Geometry check sheet. Reference: the model listing, model coordinates, mm. A direction names the side the tool comes from. Give positions to 0.01 mm unless a question says otherwise; leave off trailing zeros. Order: outer loops, then holes, each group sorted by start corner. A loop starts at its lowest first (then second) coordinate and runs counter-clockwise, first axis right, second up.
```python
from build123d import *

# Parameters (mm, degrees)
SKETCH1_R                       = 85
SKETCH1_R_2                     = 80
SKETCH1_R_3                     = 75
BOSS_EXTRUDE1_DEPTH             = 150
SKETCH1_4_R                     = 80
SKETCH1_4_R_2                   = 75
CUT_EXTRUDE1_DEPTH              = 155
SKETCH2_R                       = 85
BOSS_EXTRUDE3_DEPTH             = 5
SKETCH2_3_W                     = 20
SKETCH2_3_H                     = 96
BOSS_EXTRUDE4_DEPTH             = 176
SKETCH2_4_W                     = 20
SKETCH2_4_H                     = 96
BOSS_EXTRUDE5_DEPTH             = 176
SKETCH3_R                       = 23.5
CUT_EXTRUDE3_DEPTH              = 90
CUT_EXTRUDE4_DEPTH              = 120
CUT_EXTRUDE5_DEPTH              = 20
CUT_EXTRUDE6_START              = -20
CUT_EXTRUDE6_DEPTH              = 20
SKETCH6_R                       = 2
CUT_EXTRUDE7_DEPTH              = 20
SKETCH11_R                      = 2.5
CUT_EXTRUDE10_DEPTH             = 131
SKETCH1_7_R                     = 80
SKETCH1_7_R_2                   = 75
BOSS_EXTRUDE6_DEPTH             = 155
CUT_EXTRUDE12_DEPTH             = 20
CUT_EXTRUDE12_DEPTH_BACK        = 10
SKETCH1_10_R                    = 85
SKETCH1_10_R_2                  = 80
CUT_EXTRUDE13_START             = -25
SKETCH12_R                      = 85
SKETCH12_R_2                    = 80
CUT_EXTRUDE13_DEPTH             = 25
SKETCH1_11_R                    = 75
BOSS_EXTRUDE7_DEPTH             = 5
F_5_0MM_DOWEL_HOLE1_D           = 5
F_5_0MM_DOWEL_HOLE1_DEPTH       = 5
F_5_0MM_DOWEL_HOLE1_CSINK_D     = 5.05
F_5_0MM_DOWEL_HOLE1_CSINK_ANGLE = 90
F_5_0MM_DOWEL_HOLE1_TIP         = 1.502151548
BOSS_EXTRUDE8_DEPTH             = 3
SKETCH16_R                      = 25
CUT_EXTRUDE14_DEPTH             = 1


with BuildPart() as part:
    # Sketch1 → Boss-Extrude1 (new body)
    # profile 1 of 2: a face of its own
    with BuildSketch(Plane(origin=(0, 0, 0), x_dir=(1, 0, 0), z_dir=(0, 1, 0))):
        with Locations(Location((0, 0, 0), (0, 0, 270))):
            Circle(SKETCH1_R)
        Circle(SKETCH1_R_2, mode=Mode.SUBTRACT)
    # profile 2 of 2: a face of its own
    with BuildSketch(Plane(origin=(0, 0, 0), x_dir=(1, 0, 0), z_dir=(0, 1, 0))):
        Circle(SKETCH1_R_2)
        with Locations(Location((0, 0, 0), (0, 0, 270))):
            Circle(SKETCH1_R_3, mode=Mode.SUBTRACT)
    extrude(amount=BOSS_EXTRUDE1_DEPTH)

    # Sketch1_4 → Cut-Extrude1 (cut)
    with BuildSketch(Plane(origin=(0, 0, 0), x_dir=(1, 0, 0), z_dir=(0, 1, 0))):
        with Locations(Location((0, 0, 0), (0, 0, 270))):
            Circle(SKETCH1_4_R)
        Circle(SKETCH1_4_R_2, mode=Mode.SUBTRACT)
    extrude(amount=CUT_EXTRUDE1_DEPTH, mode=Mode.SUBTRACT)

    # Sketch2 → Boss-Extrude3 (add)
    with BuildSketch(Plane(origin=(0, 150, 0), x_dir=(1, 0, 0), z_dir=(0, 1, 0))):
        with Locations(Location((0, 0, 0), (0, 0, 270))):
            Circle(SKETCH2_R)
    extrude(amount=BOSS_EXTRUDE3_DEPTH)

    # Sketch2_3 → Boss-Extrude4 (add)
    with BuildSketch(Plane(origin=(0, 150, 0), x_dir=(1, 0, 0), z_dir=(0, 1, 0))):
        with Locations((50, 0)):
            Rectangle(SKETCH2_3_W, SKETCH2_3_H)
    extrude(amount=BOSS_EXTRUDE4_DEPTH)

    # Sketch2_4 → Boss-Extrude5 (add)
    with BuildSketch(Plane(origin=(0, 150, 0), x_dir=(1, 0, 0), z_dir=(0, 1, 0))):
        with Locations((-50, 0)):
            Rectangle(SKETCH2_4_W, SKETCH2_4_H)
    extrude(amount=BOSS_EXTRUDE5_DEPTH)

    # Sketch3 → Cut-Extrude3 (cut)
    with BuildSketch(Plane(origin=(60, 0, 0), x_dir=(0, 0, -1), z_dir=(1, 0, 0))):
        with Locations((0, 278)):
            Circle(SKETCH3_R)
    extrude(amount=-CUT_EXTRUDE3_DEPTH, mode=Mode.SUBTRACT)

    # Sketch3_3 → Cut-Extrude4 (cut)
    with BuildSketch(Plane(origin=(60, 0, 0), x_dir=(0, 0, -1), z_dir=(1, 0, 0))):
        with BuildLine():
            ThreePointArc((0, 300.5), (-22.5, 278), (0, 255.5))
            Line((0, 255.5), (0, 300.5))
        make_face()
        with BuildLine():
            Line((0, 300.5), (0, 255.5))
            ThreePointArc((0, 255.5), (15.909902577, 262.090097423), (22.5, 278))
            ThreePointArc((22.5, 278), (15.909902577, 293.909902577), (0, 300.5))
        make_face()
        with BuildLine():
            ThreePointArc((0, 301.5), (-23.5, 278), (0, 254.5))
            Line((0, 254.5), (0, 255.5))
            ThreePointArc((0, 255.5), (-22.5, 278), (0, 300.5))
            Line((0, 300.5), (0, 301.5))
        make_face()
        with BuildLine():
            Line((0, 255.5), (0, 254.5))
            ThreePointArc((0, 254.5), (16.617009358, 261.382990642), (23.5, 278))
            ThreePointArc((23.5, 278), (16.617009358, 294.617009358), (0, 301.5))
            Line((0, 301.5), (0, 300.5))
            ThreePointArc((0, 300.5), (15.909902577, 293.909902577), (22.5, 278))
            ThreePointArc((22.5, 278), (15.909902577, 262.090097423), (0, 255.5))
        make_face()
    extrude(amount=-CUT_EXTRUDE4_DEPTH, mode=Mode.SUBTRACT)

    # Sketch4 → Cut-Extrude5 (cut)
    with BuildSketch(Plane(origin=(60, 0, 0), x_dir=(0, 0, -1), z_dir=(1, 0, 0))):
        with BuildLine():
            Line((-48, 326), (-48, 278))
            ThreePointArc((-48, 278), (-33.941125268, 311.941125726), (6.48e-07, 326))
            Line((6.48e-07, 326), (-48, 326))
        make_face()
        with BuildLine():
            ThreePointArc((6.48e-07, 326), (33.941125726, 311.941125268), (48, 278))
            Line((48, 278), (48, 326))
            Line((48, 326), (6.48e-07, 326))
        make_face()
    extrude(amount=-CUT_EXTRUDE5_DEPTH, mode=Mode.SUBTRACT)

    # Sketch5 → Cut-Extrude6 (cut)
    with BuildSketch(Plane.ZY.offset(60).offset(CUT_EXTRUDE6_START)):
        with BuildLine():
            Line((-48, 326), (-48, 278))
            ThreePointArc((-48, 278), (-33.941125497, 311.941125497), (0, 326))
            Line((0, 326), (-48, 326))
        make_face()
        with BuildLine():
            ThreePointArc((0, 326), (33.941125497, 311.941125497), (48, 278))
            Line((48, 278), (48, 326))
            Line((48, 326), (0, 326))
        make_face()
    extrude(amount=CUT_EXTRUDE6_DEPTH, mode=Mode.SUBTRACT)

    # Sketch6 → Cut-Extrude7 (cut)
    with BuildSketch(Plane(origin=(60, 0, 0), x_dir=(0, 0, -1), z_dir=(1, 0, 0))):
        with Locations((0, 320)):
            Circle(SKETCH6_R)
        with Locations((29.69848481, 307.69848481)):
            Circle(SKETCH6_R)
        with Locations((42, 278)):
            Circle(SKETCH6_R)
        with Locations((29.69848481, 248.30151519)):
            Circle(SKETCH6_R)
        with Locations((0, 236)):
            Circle(SKETCH6_R)
        with Locations((-29.69848481, 248.30151519)):
            Circle(SKETCH6_R)
        with Locations((-42, 278)):
            Circle(SKETCH6_R)
        with Locations((-29.69848481, 307.69848481)):
            Circle(SKETCH6_R)
    extrude(amount=-CUT_EXTRUDE7_DEPTH, mode=Mode.SUBTRACT)

    # Sketch11 → Cut-Extrude10 (cut)
    with BuildSketch(Plane(origin=(60, 0, 0), x_dir=(0, 0, -1), z_dir=(1, 0, 0))):
        with Locations((-40, 195.5)):
            Circle(SKETCH11_R)
        with Locations((40, 195.5)):
            Circle(SKETCH11_R)
    extrude(amount=-CUT_EXTRUDE10_DEPTH, mode=Mode.SUBTRACT)

    # Sketch1_7 → Boss-Extrude6 (add)
    with BuildSketch(Plane(origin=(0, 0, 0), x_dir=(1, 0, 0), z_dir=(0, 1, 0))):
        Circle(SKETCH1_7_R)
        with Locations(Location((0, 0, 0), (0, 0, 270))):
            Circle(SKETCH1_7_R_2, mode=Mode.SUBTRACT)
    extrude(amount=BOSS_EXTRUDE6_DEPTH)

    # Sketch1_10 → Cut-Extrude12 (cut, two sides: drawn at the far end of the back side and taken through both)
    with BuildSketch(Plane(origin=(0, 0, 0), x_dir=(1, 0, 0), z_dir=(0, 1, 0)).offset(-CUT_EXTRUDE12_DEPTH_BACK)):
        with Locations(Location((0, 0, 0), (0, 0, 270))):
            Circle(SKETCH1_10_R)
        with Locations(Location((0, 0, 0), (0, 0, 270))):
            Circle(SKETCH1_10_R_2, mode=Mode.SUBTRACT)
    extrude(amount=CUT_EXTRUDE12_DEPTH + CUT_EXTRUDE12_DEPTH_BACK, mode=Mode.SUBTRACT)

    # Sketch12 → Cut-Extrude13 (cut)
    with BuildSketch(Plane(origin=(0, 155, 0), x_dir=(1, 0, 0), z_dir=(0, 1, 0)).offset(CUT_EXTRUDE13_START)):
        with Locations(Location((0, 0, 0), (0, 0, 270))):
            Circle(SKETCH12_R)
        with Locations(Location((0, 0, 0), (0, 0, 270))):
            Circle(SKETCH12_R_2, mode=Mode.SUBTRACT)
    extrude(amount=CUT_EXTRUDE13_DEPTH, mode=Mode.SUBTRACT)

    # Sketch1_11 → Boss-Extrude7 (add)
    with BuildSketch(Plane(origin=(0, 0, 0), x_dir=(1, 0, 0), z_dir=(0, 1, 0))):
        with Locations(Location((0, 0, 0), (0, 0, 270))):
            Circle(SKETCH1_11_R)
    extrude(amount=BOSS_EXTRUDE7_DEPTH)

    # 5.0mm Dowel Hole1
    with Locations(Plane(origin=(0, 0, 0), x_dir=(-1, 0, 0), z_dir=(0, -1, 0))):
        with Locations((12.340862004, 7.125), (-12.340862004, 7.125), (0, -14.25)):
            CounterSinkHole(F_5_0MM_DOWEL_HOLE1_D / 2, F_5_0MM_DOWEL_HOLE1_CSINK_D / 2, depth=F_5_0MM_DOWEL_HOLE1_DEPTH, counter_sink_angle=F_5_0MM_DOWEL_HOLE1_CSINK_ANGLE)
            with Locations((0, 0, -(F_5_0MM_DOWEL_HOLE1_DEPTH + F_5_0MM_DOWEL_HOLE1_TIP / 2))):  # 118° drill point
                Cone(0, F_5_0MM_DOWEL_HOLE1_D / 2, F_5_0MM_DOWEL_HOLE1_TIP, mode=Mode.SUBTRACT)

    # Sketch3_4 → Boss-Extrude8 (add)
    with BuildSketch(Plane(origin=(60, 0, 0), x_dir=(0, 0, -1), z_dir=(1, 0, 0))):
        with BuildLine():
            ThreePointArc((0, 301.5), (-23.5, 278), (0, 254.5))
            Line((0, 254.5), (0, 255.5))
            ThreePointArc((0, 255.5), (-22.5, 278), (0, 300.5))
            Line((0, 300.5), (0, 301.5))
        make_face()
        with BuildLine():
            Line((0, 255.5), (0, 254.5))
            ThreePointArc((0, 254.5), (16.617009358, 261.382990642), (23.5, 278))
            ThreePointArc((23.5, 278), (16.617009358, 294.617009358), (0, 301.5))
            Line((0, 301.5), (0, 300.5))
            ThreePointArc((0, 300.5), (15.909902577, 293.909902577), (22.5, 278))
            ThreePointArc((22.5, 278), (15.909902577, 262.090097423), (0, 255.5))
        make_face()
    extrude(amount=-BOSS_EXTRUDE8_DEPTH)

    # Sketch16 → Cut-Extrude14 (cut)
    with BuildSketch(Plane.ZY.offset(57)):
        with Locations((0, 278)):
            Circle(SKETCH16_R)
    extrude(amount=CUT_EXTRUDE14_DEPTH, mode=Mode.SUBTRACT)


solid = part.part
```
Q1. Gauge pin test, flat ends, axial feed: P1, Ø1, axis at x = 57, y = 90.5, coming from the -Z side; P2, Ø2, axis at x = -51.5, y = 273, coming from the +Z side; P3, Ø5, axis at y = 278, z = -42, coming from the -X side. Record the tip position at first contact, or that the pin passes through.
Q2. Cross-section at A-A, the plane y = 188.5. Record the boundary of the cut face in (x, z).
Q3. Cross-section at B-B, the plane x = 27. Record the boundary of the cut face in (y, z).
Q4. Cross-section at C-C, the plane z = 63. Record the boundary of the cut face in (x, y), and give its area (3 significant figures).
Q5. Access from +Z, -Z, +X, -X, +Y, -Y to the whole of each face (thin tool, end or side, straight path). Record for faces 1 (the face through (-60, 220, 1)), 2 (the face through (48.62, 269, -21.71)), 3 (the face through (-50, 216, -48)).
Q6. Thickness scan on L1, parallel to Z at x = 55.5, y = 278; L2, parallel to Y at x = 4.5, z = 7.5; L3, parallel to Y at x = -56, z = -19. Record the ranges inside material, lowest first.
Q7. Release check for a two-part mould opening along X. For faces 4 (the face through (-57.493, 302.787, -3.255)), 5 (the face through (-51.721, 74.23, -67.453)), 6 (the face through (1, 155, -1)), 7 (the face through (50, 216, 48)) record: pulls with the +X half, pulls with the -X half, needs draft (parallel to the pull), parting line crosses it, or undercut.
Answers follow:
1. P1: stops at z = -63.5
1. P2: stops at z = 48
1. P3: stops at x = -60
2. outline: (-60, -48) - (-40, -48) - (-40, 48) - (-60, 48) - close; (40, -48) - (60, -48) - (60, 48) - (40, 48) - close
3. outline: (0, -75.31) - (20, -75.31) - (20, -80.6) - (130, -80.6) - (130, -75.31) - (155, -75.31) - (155, 75.31) - (130, 75.31) - (130, 80.6) - (20, 80.6) - (20, 75.31) - (0, 75.31) - close; hole (5, -69.97) - (150, -69.97) - (150, 69.97) - (5, 69.97) - close
4. outline: (-57.06, 20) - (-49.31, 20) - (-49.31, 0) - (49.31, 0) - (49.31, 20) - (57.06, 20) - (57.06, 130) - (49.31, 130) - (49.31, 155) - (-49.31, 155) - (-49.31, 130) - (-57.06, 130) - close; hole (-40.69, 5) - (40.69, 5) - (40.69, 150) - (-40.69, 150) - close
4. area: 5,190 mm2
5. face 1: +Z, -Z, -X, +Y
5. face 2: -X
5. face 3: -Z, +X, -X, +Y
6. L1: z = -48 to -44, -40 to -23.5, 23.5 to 40, 44 to 48
6. L2: y = 0 to 5, 150 to 155
6. L3: y = 0 to 5, 150 to 264.17, 291.83 to 322.08
7. face 4: undercut
7. face 5: parting line crosses it
7. face 6: undercut
7. face 7: needs draft
